```python
from build123d import *

# Parameters (mm, degrees)
SKETCH1_W                                = 1150
SKETCH1_H                                = 1150
SKETCH1_W_2                              = 1118.25
SKETCH1_H_2                              = 1118.25
BOSS_EXTRUDE1_DEPTH                      = 15.875
SKETCH2_W                                = 15.875
SKETCH2_H                                = 15.875
BOSS_EXTRUDE2_DEPTH                      = 318.25
SKETCH3_W                                = 1150
SKETCH3_H                                = 1150
SKETCH3_W_2                              = 1118.25
SKETCH3_H_2                              = 1118.25
BOSS_EXTRUDE3_DEPTH                      = 15.875
BOSS_EXTRUDE4_DEPTH                      = 15.875
MIRROR2_AT_THE_SECOND_PLANE_COPY_1_DEPTH = 15.875


with BuildPart() as part:
    # Sketch1 → Boss-Extrude1 (new body)
    with BuildSketch(Plane(origin=(0, 0, 0), x_dir=(1, 0, 0), z_dir=(0, 1, 0))):
        Rectangle(SKETCH1_W, SKETCH1_H)
        Rectangle(SKETCH1_W_2, SKETCH1_H_2, mode=Mode.SUBTRACT)
    extrude(amount=BOSS_EXTRUDE1_DEPTH)

    # Sketch2 → Boss-Extrude2 (add)
    with BuildSketch(Plane(origin=(0, 15.875, 0), x_dir=(1, 0, 0), z_dir=(0, 1, 0))):
        with Locations((-567.0625, 567.0625)):
            Rectangle(SKETCH2_W, SKETCH2_H)
        with Locations((-567.0625, -567.0625)):
            Rectangle(SKETCH2_W, SKETCH2_H)
        with Locations((-567.0625, 0)):
            Rectangle(SKETCH2_W, SKETCH2_H)
    boss_extrude2 = extrude(amount=BOSS_EXTRUDE2_DEPTH)

    # Sketch3 → Boss-Extrude3 (add)
    with BuildSketch(Plane(origin=(0, 334.125, 0), x_dir=(1, 0, 0), z_dir=(0, 1, 0))):
        Rectangle(SKETCH3_W, SKETCH3_H)
        Rectangle(SKETCH3_W_2, SKETCH3_H_2, mode=Mode.SUBTRACT)
    extrude(amount=BOSS_EXTRUDE3_DEPTH)

    # Mirror1: Boss-Extrude2 across plane
    add(boss_extrude2.mirror(Plane(origin=(0, 0, 0), x_dir=(0, 0, 1), z_dir=(1, 0, 0))))

    # Sketch4 → Boss-Extrude4 (add)
    with BuildSketch(Plane.XY.offset(575)):
        Polygon((390.350320151, 11.225320151), (379.125, 0), (559.125, -180), (559.125, -307), (575, -307), (575, 0), (559.125, 0), (559.125, -157.549359697), align=None)
    boss_extrude4 = extrude(amount=-BOSS_EXTRUDE4_DEPTH)

    # Mirror2: Boss-Extrude4 across plane
    add(boss_extrude4.mirror(Plane(origin=(0, 0, 0), x_dir=(0, 0, 1), z_dir=(1, 0, 0))))

    # Mirror2 at the second plane: Boss-Extrude4 across plane
    add(boss_extrude4.mirror(Plane.XY))

    # Mirror2 at the second plane copy 1 sketc → Mirror2 at the second plane copy 1 (add)
    with BuildSketch(Plane(origin=(0, 0, -575), x_dir=(-1, 0, 0), z_dir=(0, 0, -1))):
        Polygon((390.350320151, 11.225320151), (379.125, 0), (559.125, -180), (559.125, -307), (575, -307), (575, 0), (559.125, 0), (559.125, -157.549359697), align=None)
    extrude(amount=-MIRROR2_AT_THE_SECOND_PLANE_COPY_1_DEPTH)


solid = part.part
```
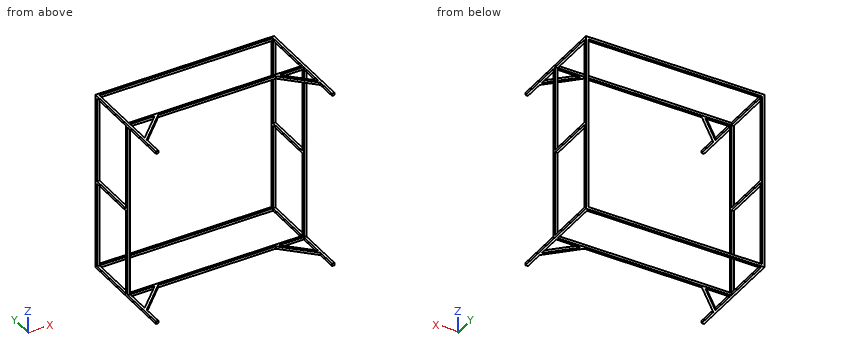
Input: part model. Units: mm. Frame: model coordinates. Coordinates: 2 decimals unless noted, no trailing zeros. Loops run counter-clockwise (first coordinate to the right, second up) from the corner with the lowest first, then second, coordinate; pieces in that order, holes last. Notation, with made-up numbers: M -18,77.25 L 27,77.25 A9 cw 27,81.25 Z; hole C -25.5,77 d10. An arc over 180 degrees is marked long. Use a Markdown table: item, result. Add a question column.
1) Section B-B, the plane z = -76.5. Return the cut outline in (x, y) (3 decimals), plus the area to 3 significant figures.
2) Section D-D, the plane x = -420.5. Return the cut outline in (y, z) (3 decimals).
3) Section C-C, the plane x = 146.5. Return the cut outline in (y, z) (3 decimals), plus the area to 3 significant figures.
4) Pin query (flat end, axial travel): P1, Ø5, axis at x = 80.5, z = -563.5, coming from the -Y side. Return the tip coordinate at first contact, or that it passes through.
5) Section A-A, the plane y = 39. Return the cut outline in (x, z) (1 decimal), plus the area to 3 significant figures.
Answer below:
| question | item | result |
|---|---|---|
| 1 | outline | M -575,0 L -559.125,0 L -559.125,15.875 L -575,15.875 Z; M -575,334.125 L -559.125,334.125 L -559.125,350 L -575,350 Z; M 559.125,0 L 575,0 L 575,15.875 L 559.125,15.875 Z; M 559.125,334.125 L 575,334.125 L 575,350 L 559.125,350 Z |
| 1 | area | 1,010 mm2 |
| 2 | outline | M -41.375,-575 L -18.924,-575 L -18.924,-559.125 L -41.375,-559.125 Z; M -41.375,559.125 L -18.924,559.125 L -18.924,575 L -41.375,575 Z; M 0,-575 L 15.875,-575 L 15.875,-559.125 L 0,-559.125 Z; M 0,559.125 L 15.875,559.125 L 15.875,575 L 0,575 Z; M 334.125,-575 L 350,-575 L 350,-559.125 L 334.125,-559.125 Z; M 334.125,559.125 L 350,559.125 L 350,575 L 334.125,575 Z |
| 3 | outline | M 0,-575 L 15.875,-575 L 15.875,-559.125 L 0,-559.125 Z; M 0,559.125 L 15.875,559.125 L 15.875,575 L 0,575 Z; M 334.125,-575 L 350,-575 L 350,-559.125 L 334.125,-559.125 Z; M 334.125,559.125 L 350,559.125 L 350,575 L 334.125,575 Z |
| 3 | area | 1,010 mm2 |
| 4 | P1 | y = 0 |
| 5 | outline | M -575,-575 L -559.1,-575 L -559.1,-559.1 L -575,-559.1 Z; M -575,-7.9 L -559.1,-7.9 L -559.1,7.9 L -575,7.9 Z; M -575,559.1 L -559.1,559.1 L -559.1,575 L -575,575 Z; M 559.1,-575 L 575,-575 L 575,-559.1 L 559.1,-559.1 Z; M 559.1,-7.9 L 575,-7.9 L 575,7.9 L 559.1,7.9 Z; M 559.1,559.1 L 575,559.1 L 575,575 L 559.1,575 Z |
| 5 | area | 1,510 mm2 |
